from build123d import *

# Parameters (mm, degrees)
SKETCH1_R           = 2.1828125
BOSS_EXTRUDE1_DEPTH = 0.79375
FILLET1_R           = 6.35


with BuildPart() as part:
    # Sketch1 → Boss-Extrude1 (new, symmetric)
    with BuildSketch(Plane.XY):
        Polygon((-28.575, 2.630256121), (-28.575, -31.75), (-19.594743879, -31.75), (-6.894743879, -19.05), (120.65, -19.05), (120.65, -10.433282549), (3.00913246, 133.35), (-6.35, 133.35), (-6.35, 24.855256121), align=None)
        Circle(SKETCH1_R, mode=Mode.SUBTRACT)
        with Locations((0, 63.5)):
            Circle(SKETCH1_R, mode=Mode.SUBTRACT)
        with Locations((12.7, -12.7)):
            Circle(SKETCH1_R, mode=Mode.SUBTRACT)
        with Locations((63.5, -12.7)):
            Circle(SKETCH1_R, mode=Mode.SUBTRACT)
        with Locations((-22.225, 0)):
            Circle(SKETCH1_R, mode=Mode.SUBTRACT)
        with Locations((-22.225, -25.4)):
            Circle(SKETCH1_R, mode=Mode.SUBTRACT)
        with Locations((0, 127)):
            Circle(SKETCH1_R, mode=Mode.SUBTRACT)
        with Locations((114.3, -12.7)):
            Circle(SKETCH1_R, mode=Mode.SUBTRACT)
    extrude(amount=BOSS_EXTRUDE1_DEPTH, both=True)

    # Fillet1
    fillet1_edges = [part.edges().sort_by_distance(p)[0] for p in [
        (120.65, -19.05, 0),
        (120.65, -10.433282549, 0),
        (-6.894743879, -19.05, 0),
        (-19.594743879, -31.75, 0),
        (-28.575, -31.75, 0),
        (-28.575, 2.630256121, 0),
        (-6.35, 24.855256121, 0),
        (3.00913246, 133.35, 0),
        (-6.35, 133.35, 0),
    ]]
    fillet(fillet1_edges, radius=FILLET1_R - 0.0001)  # a hair under: the kernel refuses the full size


solid = part.part
CAD build for the part. Positions are in the model's coordinates, mm. Coordinates: 2 decimals unless noted, no trailing zeros. Write each loop counter-clockwise with the first axis right and the second up, starting at its lowest first coordinate (ties: lowest second). Pieces come first, ordered by that corner, then holes. Notation, with made-up numbers: M 30,-3.5 L 46,-3.5 A24 ccw 46,17.5 Z; hole C 77,-28.5 d8. An arc over 180 degrees is marked long. Return JSON: item names as keys, results as strings.
Item 1: Slice it at B-B, the plane x = 12.7. Write the cut outline in (y, z), and give its area (3 significant figures).
Findings below:
{"outline": "M -19.05,-0.79 L -14.88,-0.79 L -14.88,0.79 L -19.05,0.79 Z; M -10.52,-0.79 L 121.51,-0.79 L 121.51,0.79 L -10.52,0.79 Z", "area": "216 mm2"}
Item 2: Drop a flat-ended pin along its axis: pin 1 Ø0.8 at (x, z) = (39.5, 0) entering from -Y. Give the stop position or say it passes through.
Findings below:
{"pin 1": "stops at y = -19.05"}
Item 3: Slice it at A-A, the plane z = 0.15. State how many separate pieces and enclosed holes the cut face has, and give its area (3 significant figures).
Findings below:
{"separate pieces": "1", "enclosed holes": "8", "area": "11,700 mm2"}
Item 4: Two-plate mould, pull along X, no slides. Class faces 1 (the flat face through (28, 34, 0.794)), 2 (the flat face through (62.865, 60.193, 0.011)), 3 (the cylindrical face through (61.32, -12.6, -0.01)): +X half, -X half, draft (parallel to the pull), parting line (faces both ways), or undercut.
Findings below:
{"face 1": "draft", "face 2": "+X half", "face 3": "undercut"}
Item 5: Slice it at C-C, the plane x = 63.5. Write the cut outline in (y, z).
Findings below:
{"outline": "M -19.05,-0.79 L -14.88,-0.79 L -14.88,0.79 L -19.05,0.79 Z; M -10.52,-0.79 L 59.42,-0.79 L 59.42,0.79 L -10.52,0.79 Z"}
Item 6: Slice it at D-D, the plane y = 75.5. Write the cut outline in (x, z).
Findings below:
{"outline": "M -6.35,-0.79 L 50.34,-0.79 L 50.34,0.79 L -6.35,0.79 Z"}
Item 7: Probe line 1 (Y direction, x = 0, z = 0.25); line 2 (X direction, y = -14, z = 0.4) (3 decimals); line 3 (Y direction, x = 9, z = -0.5). List the from-to ranges inside material, lowest first. Write a range as from..to.
Findings below:
{"line 1": "y = -19.05..-2.18, 2.18..61.32, 65.68..124.82, 129.18..133.35", "line 2": "x = -28.575..10.947, 14.453..61.747, 65.253..112.547, 116.053..120.516", "line 3": "y = -19.05..126.03"}
